```python
from build123d import *

# Parameters (mm, degrees)
BOSS_EXTRUDE1_DEPTH = 33.333333333
BOSS_EXTRUDE2_DEPTH = 33.333333333
CIRPATTERN2_COUNT   = 13
CIRPATTERN2_ANGLE   = 170
F_20_0MM_1_D        = 20
SCALE_1_SCALE       = 0.3
CUT_EXTRUDE_1_DEPTH = 5.5


with BuildPart() as part:
    # Sketch1 → Boss-Extrude1 (new body)
    with BuildSketch(Plane(origin=(0, 0, 0), x_dir=(1, 0, 0), z_dir=(0, 1, 0))):
        with BuildLine():
            Line((-150, 18), (-46.647615159, 18))
            ThreePointArc((-46.647615159, 18), (50, 0), (-46.647615159, -18))
            Line((-46.647615159, -18), (-150, -18))
            ThreePointArc((-150, -18), (-168, 0), (-150, 18))
        make_face()
    extrude(amount=BOSS_EXTRUDE1_DEPTH)

    # Sketch2 → Boss-Extrude2 (add)
    with BuildSketch(Plane(origin=(0, 33.333333333, 0), x_dir=(1, 0, 0), z_dir=(0, 1, 0))):
        Polygon((49.877349569, 3.5), (60, 2), (60, -2), (49.877349569, -3.5), (50, 0), align=None)
    boss_extrude2 = extrude(amount=-BOSS_EXTRUDE2_DEPTH)

    # CirPattern2: Boss-Extrude2 ×13 about axis
    cirpattern2_axis = Axis((0, 0, 0), (0, 1, 0))
    for i in range(1, CIRPATTERN2_COUNT):
        add(boss_extrude2.rotate(cirpattern2_axis, i * CIRPATTERN2_ANGLE / (CIRPATTERN2_COUNT - 1)))

    # Ø20.0mm 맞춤핀 구멍1 (through all)
    with Locations(Plane(origin=(0, 33.333333333, 0), x_dir=(1, 0, 0), z_dir=(0, 1, 0))):
        with Locations((-150, 0), (0, 0)):
            Hole(F_20_0MM_1_D / 2)


with BuildPart() as part_1:
    # 축척1: scaled about (-32.400752932, 16.666666667, -1.971262661)
    add(part.part.scale(SCALE_1_SCALE).moved(Location((-22.680527052, 11.666666667, -1.379883863))))

    # 스케치1 → 컷-돌출1 (cut)
    with BuildSketch(Plane(origin=(0, 21.666666667, 0), x_dir=(1, 0, 0), z_dir=(0, 1, 0))):
        with BuildLine():
            Line((-36.6748116, -4.020116137), (-67.680527053, -4.020116137))
            ThreePointArc((-67.680527053, -4.020116137), (-73.080527053, 1.379883863), (-67.680527053, 6.779883863))
            Line((-67.680527053, 6.779883863), (-36.6748116, 6.779883863))
            ThreePointArc((-36.6748116, 6.779883863), (-37.680527053, 1.379883863), (-36.6748116, -4.020116137))
        make_face()
    extrude(amount=-CUT_EXTRUDE_1_DEPTH, mode=Mode.SUBTRACT)


solid = part_1.part
```
Input: part model. Units: mm. Frame: model coordinates. A direction names the side the tool comes from. Coordinates: 2 decimals unless noted, no trailing zeros. Write each loop counter-clockwise with the first axis right and the second up, starting at its lowest first coordinate (ties: lowest second). Pieces come first, ordered by that corner, then holes.
1) Mould query, pull axis Z, two halves, no side actions, for faces 1 (the flat face through (-24.498, 16.737, -17.803)), 2 (the cylindrical face through (-16.06, 16.6, -14.84)), 3 (the cylindrical face through (-73.08, 13.89, -1.26)). Classes: pulls with the +Z half, pulls with the -Z half, needs draft (parallel to the pull), parting line crosses it, or undercut.
2) Material intervals for line 1 along Z through (x, y) = (-13.5, 13.75); line 2 along Y through (x, z) = (-53, -6); line 3 along Z through (x, y) = (-24, 15.25), sorted ascending.
3) Section B-B on x = -40. Output: boundary loops of the cut face in (y, z).
4) Section D-D on y = 15.5. State how many separate pieces and enclosed holes the cut face has, and give its area (3 significant figures).
5) Section C-C on z = 6.5. Output: boundary loops of the cut face in (x, y), and give its area (3 significant figures).
6) Pin query (flat end, axial travel): pin 1 Ø2.5 at (x, y) = (-53.5, 14) entering from +Z; pin 2 Ø6 at (x, z) = (-39.5, -12.5) entering from +Y; pin 3 Ø1.5 at (y, z) = (14.5, 9.5) entering from -X; pin 4 Ø6 at (y, z) = (19, 8.5) entering from -X. Return the tip coordinate at first contact, or that it passes through.
7) Section A-A on x = -67. Output: boundary loops of the cut face in (y, z), and give its area (3 significant figures).
8) Set-up query: faces 4 (the flat face through (-6.92, 16.74, -6.21)), 5 (the flat face through (-5.23, 16.74, -5.79)), 6 (the flat face through (-9.96, 16.74, -11.92)), 7 (the flat face through (-23, 21.667, 2)), 8 (the cylindrical face through (-19.55, 16.6, -16.05)). Return all of +Z, -Z, +X, -X, +Y, -Y with unobstructed straight access to the full face (end or side cutting, diameter ignored); none if empty.
Check result:
1. face 1: pulls with the -Z half
1. face 2: undercut
1. face 3: parting line crosses it
2. line 1: z = -16.51 to -13.48, -13.24 to 10.48
2. line 2: y = 11.67 to 16.17
2. line 3: z = -16.32 to -4.07, 1.31 to 13.56
3. outline: (11.67, -6.78) - (16.17, -6.78) - (16.17, 4.02) - (11.67, 4.02) - close
4. separate pieces: 1
4. enclosed holes: 2
4. area: 1,080 mm2
5. outline: (-35.44, 11.67) - (-9.92, 11.67) - (-9.92, 21.67) - (-35.44, 21.67) - close
5. area: 255 mm2
6. pin 1: stops at z = 4.02
6. pin 2: stops at y = 21.67
6. pin 3: stops at x = -33.74
6. pin 4: stops at x = -36.01
7. outline: (11.67, -6.78) - (16.17, -6.78) - (16.17, -4.3) - (11.67, -4.3) - close; (11.67, 1.54) - (16.17, 1.54) - (16.17, 4.02) - (11.67, 4.02) - close
7. area: 22.3 mm2
8. face 4: +Y, -Y
8. face 5: -Z, +X, +Y, -Y
8. face 6: +X, +Y, -Y
8. face 7: +Z, -Z, +X, -X, +Y
8. face 8: -Z, +Y, -Y
